Source: CAD feature listing. Evaluate the final solid. Frame: model axes, mm. Give positions to 0.01 mm unless a question says otherwise; leave off trailing zeros. Order: outer loops, then holes, each group sorted by start corner. A loop starts at its lowest first (then second) coordinate and runs counter-clockwise, first axis right, second up. Notation, with made-up numbers: M 21.5,53.25 L 40.5,53.25 A27 ccw 40.5,91.25 Z; hole C 5.25,32 d10. An arc over 180 degrees is marked long. Use CSV: the item, a comma, the result in double quotes. Start each with the question number.
Item 1: Section query D-D on y = 0.9. Count the separate pieces of the cut face and the enclosed holes in it, and give its area (3 significant figures).
Item 2: Section query B-B on x = 1.7. Return loops of the section in (y, z), and give its area (3 significant figures).
Item 3: Section query A-A on y = 0. Return loops of the section in (x, z), and give its area (3 significant figures).
Item 4: First-contact query: pin 1 (1.5 mm diameter, centred on y = 0, z = 2, fed in from -X); pin 2 (2 mm diameter, centred on x = -1, y = -1, fed in from +Z); pin 3 (2.5 mm diameter, centred on x = 0, y = 0, fed in from +Z); pin 4 (2.5 mm diameter, centred on y = 0, z = 2.5, fed in from +X). Flat tips, straight axial feed; report the tip coordinate or a pass-through.
Item 5: Ray query, probe 1 along Y at (x, z) = (1.1, 2.5); probe 2 along Y at (x, z) = (-1.15, 1.65). Return the intervals inside material, ascending. Write a range as from..to.
Item 6: Section query C-C on z = 4.35. Return loops of the section in (x, y).
Item 7: Pull-direction query (X, two-part tool) for faces 1 (the face through (0, -2.5, 2)), 2 (the face through (2.5, -1.4, 3.4)), 3 (the face through (1, 0, 4)); classes: +X half, -X half, draft (parallel to the pull), parting line (faces both ways), or undercut.
from build123d import *

# Parameters (mm, degrees)
ESQUISSE1_W             = 5
ESQUISSE1_H             = 5
ESQUISSE1_R             = 1
BOSS_EXTRU_1_DEPTH      = 5
ESQUISSE2_R             = 1
ENL_V_MAT_EXTRU_1_DEPTH = 10
CONG_1_R                = 0.5


with BuildPart() as part:
    # Esquisse1 → Boss.-Extru.1 (new body)
    with BuildSketch(Plane.XY):
        Rectangle(ESQUISSE1_W, ESQUISSE1_H)
        Circle(ESQUISSE1_R, mode=Mode.SUBTRACT)
    extrude(amount=BOSS_EXTRU_1_DEPTH)

    # Esquisse2 → Enlèv. mat.-Extru.1 (cut)
    with BuildSketch(Plane(origin=(2.5, 0, 0), x_dir=(0, 0, -1), z_dir=(1, 0, 0))):
        with Locations((-2.5, 0)):
            Circle(ESQUISSE2_R)
    extrude(amount=-ENL_V_MAT_EXTRU_1_DEPTH, mode=Mode.SUBTRACT)

    # Congé1
    cong_1_edges = [part.edges().sort_by_distance(p)[0] for p in [
        (-2.5, 0, 5),
        (-1, 0, 0),
        (-1, 0, 5),
        (0, -2.5, 5),
        (-2.5, 0, 3.5),
        (2.5, 0, 3.5),
        (2.5, 0, 5),
        (0, -2.5, 0),
        (-2.5, 0, 0),
        (0, 2.5, 0),
        (2.5, 0, 0),
        (0, 2.5, 5),
        (2.5, -2.5, 2.5),
        (-2.5, -2.5, 2.5),
        (-2.5, 2.5, 2.5),
        (2.5, 2.5, 2.5),
    ]]
    fillet(cong_1_edges, radius=CONG_1_R)


solid = part.part
Verdict:
1,separate pieces,"4"
1,enclosed holes,"0"
1,area,"16.1 mm2"
2,outline,"M -2.5,0.5 A0.5 ccw -2,0 L 2,0 A0.5 ccw 2.5,0.5 L 2.5,4.5 A0.5 ccw 2,5 L -2,5 A0.5 ccw -2.5,4.5 Z; hole C 0,2.5 d2"
2,area,"21.6 mm2"
3,outline,"M -2.5,0.5 A0.5 ccw -2,0 L -1.5,0 A0.5 ccw -1,0.5 L -1,1.5 L -2,1.5 A0.5 ccw -2.5,1 Z; M -2.5,4 A0.5 ccw -2,3.5 L -1,3.5 L -1,4.5 A0.5 ccw -1.5,5 L -2,5 A0.5 ccw -2.5,4.5 Z; M 1,0.5 A0.5 ccw 1.5,0 L 2,0 A0.5 ccw 2.5,0.5 L 2.5,1 A0.5 ccw 2,1.5 L 1,1.5 Z; M 1,3.5 L 2,3.5 A0.5 ccw 2.5,4 L 2.5,4.5 A0.5 ccw 2,5 L 1.5,5 A0.5 ccw 1,4.5 Z"
3,area,"8.36 mm2"
4,pin 1,"x = -2.43"
4,pin 2,"z = 5"
4,pin 3,"z = 4.93"
4,pin 4,"x = 2.43"
5,probe 1,"-2.5..-1, 1..2.5"
5,probe 2,"-2.5..-0.53, 0.53..2.5"
6,outline,"M -2.5,-2 A0.5 ccw -2,-2.5 L 2,-2.5 A0.5 ccw 2.5,-2 L 2.5,2 A0.5 ccw 2,2.5 L -2,2.5 A0.5 ccw -2.5,2 Z; hole C 0,0 d2"
7,face 1,"draft"
7,face 2,"+X half"
7,face 3,"undercut"
